Check sheet for the modelled part. Datum: model origin and axes. Units: mm. A direction names the side the tool comes from. Round coordinates to 2 decimals unless told otherwise and drop trailing zeros. Write each loop counter-clockwise with the first axis right and the second up, starting at its lowest first coordinate (ties: lowest second). Pieces come first, ordered by that corner, then holes.
Item 1: Cross-section at A-A on z = 17.5. Enter the section's corners in (x, y), plus the area to 3 significant figures.
Item 2: Tool access check on faces 5 (the flat face through (44, -19.05, 19)), 6 (the flat face through (19.215, -15.653, 19.139)), 7 (the flat face through (25, -16, 0)). Record the directions out of +Z, -Z, +X, -X, +Y, -Y that give a thin tool (end or side, any length) a straight path to the whole face; none if there is none.
Item 3: Release check for a two-part mould opening along X. For faces 1 (the flat face through (44, -25, 25.4)), 2 (the flat face through (50.769, -25, 19)), 3 (the flat face through (38.1, -25, 19)), 4 (the flat face through (0, -16, 13)) record: +X half, -X half, draft (parallel to the pull), parting line (faces both ways), or undercut.
Item 4: Material ranges on line 1 (Z direction, x = 41, y = -8); line 2 (Y direction, x = 42.5, z = 22.5); line 3 (X direction, y = -28, z = 24.25), recorded low to high.
Item 5: Cross-section at D-D on y = -13. Enter the section's corners in (x, z).
Item 6: Go/stop test with flat-tipped pins: pin 1 Ø10 at (y, z) = (-27, 19.5) entering from +X; pin 2 Ø4 at (x, z) = (41.5, 20) entering from -Y; pin 3 Ø3.5 at (x, z) = (44, 18) entering from +Y. Record where each tip stops, or that it passes through.
from build123d import *

# Parameters (mm, degrees)
F0_W     = 50.8
F0_H     = 25.4
F1_DEPTH = 31.75
F2_W     = 19.05
F2_H     = 12.7
F3_DEPTH = 19.05
F6_DEPTH = 12.7


with BuildPart() as f1:
    # F0 (on Front) → F1 (new body)
    with BuildSketch(Plane.XZ):
        with Locations((25.4, 12.7)):
            Rectangle(F0_W, F0_H)
    extrude(amount=F1_DEPTH)

    # F2 (on face) → F3 (cut)
    with BuildSketch(Plane.YZ.offset(50.8)):
        with Locations((-9.525, 19.05)):
            Rectangle(F2_W, F2_H)
    extrude(amount=-F3_DEPTH, mode=Mode.SUBTRACT)

    # F5 (on face) → F6 (cut)
    with BuildSketch(Plane.XY.offset(25.4)):
        Polygon((50.768599, -31.724313), (38.1, -31.724313), (38.1, -19.05), (31.75, -19.05), (31.75, 0), (6.32382, -31.75), (50.8, -31.75), (50.8, -19.05), (50.347392, -19.05), (50.768599, -19.064216), align=None)
    extrude(amount=-F6_DEPTH, mode=Mode.SUBTRACT)


solid = f1.part
Response values:
1. outline: (0, -31.75) - (6.32, -31.75) - (31.75, 0) - (0, 0) - close; (38.1, -31.72) - (50.77, -31.72) - (50.77, -19.06) - (50.35, -19.05) - (38.1, -19.05) - close
1. area: 765 mm2
2. face 5: +Z, +X, +Y
2. face 6: +Z, -Y
2. face 7: -Z, +X, -X, +Y, -Y
3. face 1: draft
3. face 2: +X half
3. face 3: undercut
3. face 4: -X half
4. line 1: z = 0 to 12.7
4. line 2: y = -31.72 to -19.05
4. line 3: x = 0 to 9.33, 38.1 to 50.77
5. outline: (0, 0) - (50.8, 0) - (50.8, 12.7) - (21.34, 12.7) - (21.34, 25.4) - (0, 25.4) - close
6. pin 1: stops at x = 50.77
6. pin 2: stops at y = -31.72
6. pin 3: stops at y = -19.05
